Could you check a few things on this model? Use its own coordinates, in mm. A direction names the side the tool comes from. Give positions to 0.01 mm unless a question says otherwise; leave off trailing zeros. Order: outer loops, then holes, each group sorted by start corner. A loop starts at its lowest first (then second) coordinate and runs counter-clockwise, first axis right, second up. Notation, with made-up numbers: M 15.5,59.25 L 24.5,59.25 A18 cw 24.5,64.25 Z; hole C 47.5,16 d3. An arc over 180 degrees is marked long. Use a Markdown table: item, result. Add a question column.
Item 1: Suppose I cut it at B-B on x = 11.5. Write out the boundary of the cut face in (y, z).
Item 2: If we mould it in two halves opening along Z, with no side actions, what happens to faces 1 (the face through (75, 49, 125)), 2 (the face through (20, 95, -120)), 3 (the face through (12.675, 31.574, -8.104)), 4 (the face through (13, 30, 35))? For each: released by +Z, released by -Z, zero draft, split by the parting line, or undercut.
Item 3: For faces 5 (the face through (-1.953, 35.128, -84.86)), 6 (the face through (0, 50, -25)), 7 (the face through (0, 5, -100)), 8 (the face through (0, 50, 125)), which set-ups out of +Z, -Z, +X, -X, +Y, -Y let a thin tool reach every point of the face, with its end or its side?
Item 4: If I drill on L1, parallel to Z at x = 16.5, y = 50; L2, parallel to Y at x = -19.5, z = -93.5; L3, parallel to X at y = 55.5, z = -83, over which ranges is the centre line in solid material (lowest first)? Write a range as from..to.
Item 5: I'm going to push flat-ended pins straight in: pin 1 Ø25 at (y, z) = (49, 50.5) entering from +X; pin 2 Ø11 at (x, y) = (6.5, 95.5) entering from -Z; pin 3 Ø10 at (x, y) = (-3, 21) entering from -Z. Where does each tip first touch, or does it pass through?
Item 6: Suppose I cut it at A-A on z = 50. Write out the boundary of the cut face in (x, y).
Item 7: Suppose I cut it at C-C on y = 50. Write out the boundary of the cut face in (x, z).
Item 8: Suppose I cut it at D-D on x = 52. Write out the boundary of the cut face in (y, z), plus the area to 3 significant figures.
from build123d import *

# Parameters (mm, degrees)
F1_DEPTH  = 100
F2_R      = 25
F3_DEPTH  = 25
F5_W      = 40
F5_H      = 80
F6_DEPTH  = 25
F7_R      = 15
F8_DEPTH  = 20
F10_DEPTH = 20
F11_W     = 50
F11_H     = 50
F12_DEPTH = 25


with BuildPart() as f1:
    # F0 (on Front) → F1 (new body)
    with BuildSketch(Plane.XZ):
        Polygon((-25, -100), (25, -100), (25, 100), (75, 100), (75, 150), (-25, 150), (-25, 100), align=None)
    extrude(amount=-F1_DEPTH)

    # F2 (on face) → F3 (cut)
    with BuildSketch(Plane.YZ.offset(25)):
        with Locations((50, -25)):
            Circle(F2_R)
        with Locations((50, 50)):
            Circle(F2_R)
    extrude(amount=-F3_DEPTH, mode=Mode.SUBTRACT)

    # F5 (on face) → F6 (cut)
    with BuildSketch(Plane(origin=(0, 0, -100), x_dir=(1, 0, 0), z_dir=(0, 0, -1))):
        with Locations((0, -50)):
            Rectangle(F5_W, F5_H)
    extrude(amount=-F6_DEPTH, mode=Mode.SUBTRACT)

    # F7 (on face) → F8 (join)
    with BuildSketch(Plane(origin=(0, 0, -75), x_dir=(1, 0, 0), z_dir=(0, 0, -1))):
        with Locations((0, -50)):
            Circle(F7_R)
    extrude(amount=F8_DEPTH)

    # F9 (on face) → F10 (join)
    with BuildSketch(Plane(origin=(0, 0, -100), x_dir=(1, 0, 0), z_dir=(0, 0, -1))):
        Polygon((-25, -10), (-20, -10), (-15, -10), (-15, 0), (-25, 0), align=None)
        Polygon((20, -10), (25, -10), (25, 0), (15, 0), (15, -10), align=None)
        Polygon((15, -100), (25, -100), (25, -90), (20, -90), (15, -90), align=None)
        Polygon((-25, -100), (-15, -100), (-15, -90), (-20, -90), (-25, -90), align=None)
    extrude(amount=F10_DEPTH)

    # F11 (on face) → F12 (cut)
    with BuildSketch(Plane(origin=(-25, 0, 0), x_dir=(0, -1, 0), z_dir=(-1, 0, 0))):
        with Locations((-50, 125)):
            Rectangle(F11_W, F11_H)
    extrude(amount=-F12_DEPTH, mode=Mode.SUBTRACT)


solid = f1.part
Findings below:
| question | item | result |
|---|---|---|
| 1 | outline | M 0,-100 L 10,-100 L 10,-75 L 40.37,-75 L 40.37,-95 L 59.63,-95 L 59.63,-75 L 90,-75 L 90,-100 L 100,-100 L 100,150 L 0,150 Z; hole C 50,-25 d50; hole C 50,50 d50 |
| 2 | face 1 | zero draft |
| 2 | face 2 | released by -Z |
| 2 | face 3 | undercut |
| 2 | face 4 | undercut |
| 3 | face 5 | -Z |
| 3 | face 6 | +X |
| 3 | face 7 | -Z, +Y, -Y |
| 3 | face 8 | +Z, -X |
| 4 | L1 | z = -75..-50, 0..25, 75..150 |
| 4 | L2 | y = 0..10, 90..100 |
| 4 | L3 | x = -25..-20, -13.96..13.96, 20..25 |
| 5 | pin 1 | stops at x = 0 |
| 5 | pin 2 | stops at z = -100 |
| 5 | pin 3 | stops at z = -75 |
| 6 | outline | M -25,0 L 25,0 L 25,25 L 0,25 L 0,75 L 25,75 L 25,100 L -25,100 Z |
| 7 | outline | M -25,-100 L -20,-100 L -20,-75 L -15,-75 L -15,-95 L 15,-95 L 15,-75 L 20,-75 L 20,-100 L 25,-100 L 25,-50 L 0,-50 L 0,0 L 25,0 L 25,25 L 0,25 L 0,75 L 25,75 L 25,100 L 75,100 L 75,150 L 0,150 L 0,100 L -25,100 Z |
| 8 | outline | M 0,100 L 100,100 L 100,150 L 0,150 Z |
| 8 | area | 5,000 mm^2 |
